Model file for the job. Use its own axes, mm. A direction names the side the tool comes from. Round coordinates to 2 decimals unless told otherwise and drop trailing zeros. Order: outer loops, then holes, each group sorted by start corner. A loop starts at its lowest first (then second) coordinate and runs counter-clockwise, first axis right, second up. Notation, with made-up numbers: (-37, -32.5) -> (3, -32.5) arc R22 ccw to (3, -13.5) -> close; hole circle Ø3 at (72, -2). An arc over 180 degrees is marked (long way). Use CSV: the item, a comma, the result in double quotes.
```python
from build123d import *

# Parameters (mm, degrees)
SKETCH_W          = 40
SKETCH_H          = 23
PAD_DEPTH         = 20
SKETCH001_W       = 35
SKETCH001_H       = 18
POCKET_DEPTH      = 0.001
POCKET_DEPTH_BACK = 20.001
SKETCH002_R       = 2.75
POCKET001_DEPTH   = 3.5
SKETCH003_R       = 2
POCKET002_DEPTH   = 2.5
CHAMFER_SIZE      = 2.485
FILLET_R          = 1
FILLET001_R       = 1


with BuildPart() as part:
    # Sketch → Pad (new body)
    with BuildSketch(Plane.XZ):
        Rectangle(SKETCH_W, SKETCH_H)
    extrude(amount=PAD_DEPTH)

    # Sketch001 → Pocket (cut, two sides)
    with BuildSketch(Plane.XZ) as pocket_sk:
        Rectangle(SKETCH001_W, SKETCH001_H)
    extrude(amount=-POCKET_DEPTH, mode=Mode.SUBTRACT)
    extrude(pocket_sk.sketch, amount=POCKET_DEPTH_BACK, mode=Mode.SUBTRACT)

    # Sketch002 (on DatumPlane) → Pocket001 (cut)
    with BuildSketch(Plane(origin=(0, 0, 11.5), x_dir=(-1, 0, 0), z_dir=(0, 0, 1))):
        with Locations((-9.375, 10)):
            Circle(SKETCH002_R)
        with Locations((9.375, 10)):
            Circle(SKETCH002_R)
    extrude(amount=-POCKET001_DEPTH, mode=Mode.SUBTRACT)

    # Sketch003 (on DatumPlane) → Pocket002 (cut)
    with BuildSketch(Plane(origin=(0, 0, -9), x_dir=(-1, 0, 0), z_dir=(0, 0, 1))):
        with Locations((-9.375, 10)):
            Circle(SKETCH003_R)
        with Locations((9.375, 10)):
            Circle(SKETCH003_R)
    extrude(amount=-POCKET002_DEPTH, mode=Mode.SUBTRACT)

    # Chamfer
    chamfer_edges = [part.edges().sort_by_distance(p)[0] for p in [
        (-7.375, -10, -9),
        (11.375, -10, -9),
    ]]
    chamfer(chamfer_edges, length=CHAMFER_SIZE)

    # Fillet
    fillet_edges = [part.edges().sort_by_distance(p)[0] for p in [
        (-20, -20, 0),
        (0, -20, 11.5),
        (0, -20, -11.5),
        (20, -20, 0),
        (-17.5, -20, 0),
        (0, -20, 9),
        (17.5, -20, 0),
        (0, -20, -9),
        (-20, 0, 0),
        (0, 0, 11.5),
        (0, 0, -11.5),
        (20, 0, 0),
        (-17.5, 0, 0),
        (0, 0, 9),
        (17.5, 0, 0),
        (0, 0, -9),
        (-20, -10, 11.5),
        (20, -10, 11.5),
        (-20, -10, -11.5),
        (20, -10, -11.5),
    ]]
    fillet(fillet_edges, radius=FILLET_R)

    # Fillet001
    fillet001_edges = [part.edges().sort_by_distance(p)[0] for p in [
        (-6.625, -10, 11.5),
        (12.125, -10, 11.5),
    ]]
    fillet(fillet001_edges, radius=FILLET001_R)


solid = part.part
```
Q1. Cut at B-B (x = 2.5). Give the cut face in (y, z).
From the geometry:
outline,"(-20, -10.5) arc R1 ccw to (-19, -11.5) -> (-1, -11.5) arc R1 ccw to (0, -10.5) -> (0, -10) arc R1 ccw to (-1, -9) -> (-19, -9) arc R1 ccw to (-20, -10) -> close; (-20, 10) arc R1 ccw to (-19, 9) -> (-1, 9) arc R1 ccw to (0, 10) -> (0, 10.5) arc R1 ccw to (-1, 11.5) -> (-19, 11.5) arc R1 ccw to (-20, 10.5) -> close"
Q2. Probe line 1 along X through (y, z) = (-10, 9.6) (3 decimals); line 2 along X through (y, z) = (-5, 2.75); line 3 along Z through (x, y) = (-15.5, -5). List the from-to ranges inside material, lowest first.
From the geometry:
line 1,"x = -20 to -12.125, -6.625 to 6.625, 12.125 to 20"
line 2,"x = -20 to -17.5, 17.5 to 20"
line 3,"z = -11.5 to -9, 9 to 11.5"
Q3. Which spindle directions (+Z, -Z, +X, -X, +Y, -Y) get a long thin tool onto all of the face, cutting with end or side? Do faces 5 (the cylindrical face through (-17.801, -19.715, -0.14)), 6 (the conical face through (8.38, -8.09, -11.33)), 7 (the flat face through (-17.5, -10, 0)), 8 (the cylindrical face through (-17.801, -0.285, 0.14)). Say none if no direction does.
From the geometry:
face 5,"-Y"
face 6,"none"
face 7,"+Y, -Y"
face 8,"+Y"
Q4. Cut at C-C (y = -4.25). Give the cut face in (x, z), plus the area to 3 significant figures.
From the geometry:
outline,"(-20, -10.5) arc R1 ccw to (-19, -11.5) -> (19, -11.5) arc R1 ccw to (20, -10.5) -> (20, 10.5) arc R1 ccw to (19, 11.5) -> (-19, 11.5) arc R1 ccw to (-20, 10.5) -> close; hole (-17.5, -9) -> (17.5, -9) -> (17.5, 9) -> (-17.5, 9) -> close"
area,"289 mm²"
Q5. Mould opens along Z. For faces 1 (the cylindrical face through (-0.259, -19.699, -9.285)), 2 (the cylindrical face through (0.266, -19.699, -11.215)), 3 (the flat face through (0, -10, 11.5)), 4 (the cylindrical face through (-19.715, -19.699, 0.147)) say: +Z half, -Z half, draft (parallel to the pull), parting line (faces both ways), or undercut.
From the geometry:
face 1,"undercut"
face 2,"-Z half"
face 3,"+Z half"
face 4,"draft"
Q6. Cut at D-D (y = -10). State how many separate pieces and enclosed holes the cut face has, plus the area to 3 significant figures.
From the geometry:
separate pieces,"4"
enclosed holes,"0"
area,"228 mm²"
Q7. Cut at A-A (z = -5.5). Give the cut face in (x, y), plus the area to 3 significant figures.
From the geometry:
outline,"(-20, -19) arc R1 ccw to (-19, -20) -> (-18.5, -20) arc R1 ccw to (-17.5, -19) -> (-17.5, -1) arc R1 ccw to (-18.5, 0) -> (-19, 0) arc R1 ccw to (-20, -1) -> close; (17.5, -19) arc R1 ccw to (18.5, -20) -> (19, -20) arc R1 ccw to (20, -19) -> (20, -1) arc R1 ccw to (19, 0) -> (18.5, 0) arc R1 ccw to (17.5, -1) -> close"
area,"98.3 mm²"
